Drawing for the job (mm, zero at the part's lowest x, y, z). A direction names the side the tool comes from. Round coordinates to 2 decimals unless told otherwise and drop trailing zeros. Write each loop counter-clockwise with the first axis right and the second up, starting at its lowest first coordinate (ties: lowest second). Pieces come first, ordered by that corner, then holes. Notation, with made-up numbers: M 17,45 L 74,45 A31 cw 74,73 Z; hole C 21.5,-9.75 d9. An arc over 180 degrees is marked long. Use a Markdown table: item, result. Add a question column.
1) Slice it at D-D on z = 20. Write the cut outline in (x, y).
2) Slice it at A-A on y = 32.5. Write the cut outline in (x, z).
3) Slice it at B-B on x = 47. Write the cut outline in (y, z).
4) Which spindle directions (+Z, -Z, +X, -X, +Y, -Y) get a long thin tool onto all of the face, cutting with end or side? Do the marked faces 1 and 2. Say none if no direction does.
5) Two-plate mould, pull along Y, no slides. Class the marked faces 3, 4, 5 and 6: released by +Y, released by -Y, zero draft, split by the parting line, or undercut.
6) Drop flat-ended pins along their axis: P1, Ø3, axis at x = 35, y = 49, coming from the -Z side; P2, Ø0.5, axis at x = 10, y = 64.5, coming from the +Z side; P3, Ø10, axis at x = 35.5, y = 34, coming from the +Z side. Give the stop position or say it passes through.
7) Wall check: probe 1 along Y at (x, z) = (23, 6.5); probe 2 along Y at (x, z) = (9, 4.5); probe 3 along X at (y, z) = (44, 38.5). Give the ranges that are in metal, low to high.
8) Slice it at C-C on z = 28. Write the cut outline in (x, y), plus the area to 3 significant figures.
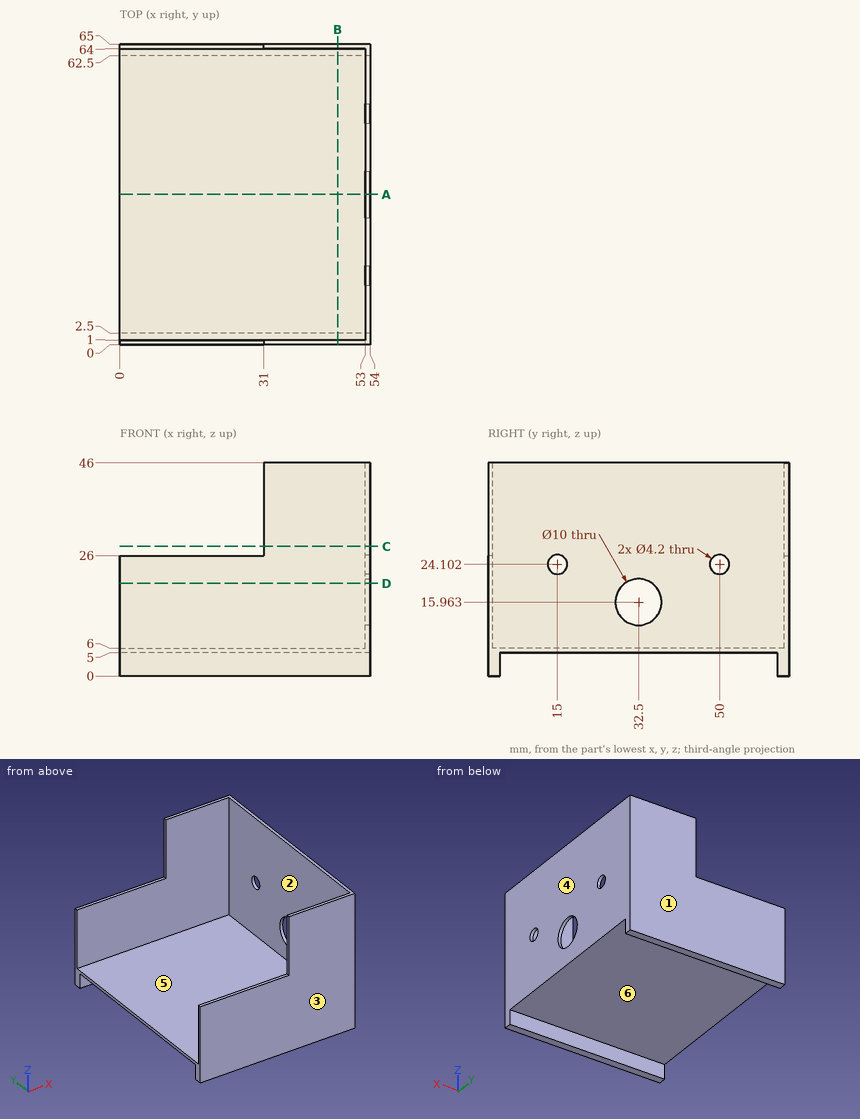
Entries:
| question | item | result |
|---|---|---|
| 1 | outline | M 0,0 L 54,0 L 54,29.55 L 53,29.55 L 53,1 L 0,1 Z; M 0,64 L 53,64 L 53,35.45 L 54,35.45 L 54,65 L 0,65 Z |
| 2 | outline | M 0,5 L 54,5 L 54,10.96 L 53,10.96 L 53,6 L 0,6 Z; M 53,20.96 L 54,20.96 L 54,46 L 53,46 Z |
| 3 | outline | M 0,0 L 2.5,0 L 2.5,5 L 62.5,5 L 62.5,0 L 65,0 L 65,46 L 64,46 L 64,6 L 1,6 L 1,46 L 0,46 Z |
| 4 | face 1 | +Z, -Z, +X, -X, +Y |
| 4 | face 2 | +Z, -X |
| 5 | face 3 | released by -Y |
| 5 | face 4 | zero draft |
| 5 | face 5 | undercut |
| 5 | face 6 | undercut |
| 6 | P1 | stops at z = 5 |
| 6 | P2 | stops at z = 26 |
| 6 | P3 | stops at z = 6 |
| 7 | probe 1 | y = 0 to 1, 64 to 65 |
| 7 | probe 2 | y = 0 to 2.5, 62.5 to 65 |
| 7 | probe 3 | x = 53 to 54 |
| 8 | outline | M 31,0 L 54,0 L 54,65 L 31,65 L 31,64 L 53,64 L 53,1 L 31,1 Z |
| 8 | area | 109 mm^2 |
